```python
from build123d import *

# Parameters (mm, degrees)
F1_DEPTH = 12
F2_DEPTH = 25
F3_R     = 2.5
F4_DEPTH = 25


# Not quite as in the source:
# - a feature names something its author has since deleted; it is built from what else it names


with BuildPart() as f1:
    # F0 (on Top) → F1 (new body)
    with BuildSketch(Plane.XY):
        with BuildLine():
            Line((5, 0), (0, -5))
            Line((0, -5), (0, -30))
            Line((0, -30), (0, -35))
            Line((0, -35), (0, -60))
            Line((0, -60), (0, -65))
            Line((0, -65), (0, -100))
            Line((0, -100), (17.4887780242, -90.9055213439))
            Line((17.4887780242, -90.9055213439), (17.4887780242, -46.2056212127))
            Line((17.4887780242, -46.2056212127), (17.4887780242, -29))
            Line((17.4887780242, -29), (17.4887780242, -20.1109461486))
            Line((17.4887780242, -20.1109461486), (57.2072267532, -20.1109461486))
            Line((57.2072267532, -20.1109461486), (65.1114210486, -29))
            Line((65.1114210486, -29), (132.5, -29))
            ThreePointArc((132.5, -29), (144.1672618896, -24.1672618896), (149, -12.5))
            Line((149, -12.5), (150, 0))
            Line((150, 0), (145.9653675556, 0))
            Line((145.9653675556, 0), (145, -1.1582256993))
            Line((145, -1.1582256993), (145, -3.3333333333))
            Line((145, -3.3333333333), (145, -12.5))
            ThreePointArc((145, -12.5), (132.5, -25), (120, -12.5))
            Line((120, -12.5), (120, -2))
            Line((120, -2), (118, 0))
            Line((118, 0), (97, 0))
            Line((97, 0), (95, -2))
            Line((95, -2), (95, -12.5))
            ThreePointArc((95, -12.5), (82.5, -25), (70, -12.5))
            Line((70, -12.5), (70, -2))
            Line((70, -2), (68, 0))
            Line((68, 0), (5, 0))
        make_face()
    extrude(amount=F1_DEPTH)

    # F0 (on Top) → F2 (cut)
    with BuildSketch(Plane.XY):
        Polygon((17.4887780242, -46.2056212127), (17.4887780242, -90.9055213439), (27.4864036634, -85.7065764627), (108.4292656183, -38.1771444678), (132.5, -29), (65.1114210486, -29), (57.2072267532, -29), (57.2072267532, -46.2056212127), align=None)
    extrude(amount=-F2_DEPTH, mode=Mode.SUBTRACT)

    # F3 (on face) → F4 (cut)
    with BuildSketch(Plane(origin=(0, 0, 0), x_dir=(0, -1, 0), z_dir=(-1, 0, 0))):
        with Locations((25, 6)):
            Circle(F3_R)
        with Locations((50, 6)):
            Circle(F3_R)
    extrude(amount=-F4_DEPTH, mode=Mode.SUBTRACT)


solid = f1.part
```
CAD build for the part. Positions are in the model's coordinates, mm. A direction names the side the tool comes from. Round coordinates to 2 decimals unless told otherwise and drop trailing zeros. Order: outer loops, then holes, each group sorted by start corner. A loop starts at its lowest first (then second) coordinate and runs counter-clockwise, first axis right, second up.
Item 1: Saw through at C-C on y = -11. Write the cut outline in (x, z), then the cut area to 3 significant figures.
Item 2: Pin check, flat tips, straight feed: pin 1 (4 mm diameter, centred on x = 94.5, z = 10, fed in from +Y); pin 2 (2 mm diameter, centred on x = 21, z = 5, fed in from -Y); pin 3 (3 mm diameter, centred on y = -18, z = 7.5, fed in from +X). Stop position of each tip, or through.
Item 3: Probe line 1 along X through (y, z) = (-13, 5); line 2 along X through (y, z) = (-9, 1.75); line 3 along Z through (x, y) = (12.5, -50). List the from-to ranges inside material, lowest first.
Item 4: Mould opens along Z. For faces 1 (the face through (8.622, -52.385, 6.751)), 2 (the face through (144.038, -24.295, 5.916)), 3 (the face through (58, -20, 0)) say: pulls with the +Z half, pulls with the -Z half, needs draft (parallel to the pull), parting line crosses it, or undercut.
Item 5: Saw through at A-A on z = 6. State how many separate pieces and enclosed holes the cut face has, then the cut area to 3 significant figures.
Item 6: Tool access for faces 4 (the face through (8.62, -23.16, 7.69)), 5 (the face through (70, -7, 6)), 6 (the face through (37, -20.111, 6)), 7 (the face through (98, -29, 6)): list every direction of +Z, -Z, +X, -X, +Y, -Y with a clear straight run to the whole face (end or side of a thin tool).
Item 7: Saw through at D-D on x = 108.5. Write the cut outline in (y, z), then the cut area to 3 significant figures.
Item 8: Saw through at B-B on y = -50. Write the cut outline in (x, z), then the cut area to 3 significant figures.
Reported:
1. outline: (0, 0) - (70, 0) - (70, 12) - (0, 12) - close; (95, 0) - (120, 0) - (120, 12) - (95, 12) - close; (145, 0) - (149.12, 0) - (149.12, 12) - (145, 12) - close
1. area: 1,190 mm2
2. pin 1: stops at y = -0.5
2. pin 2: stops at y = -20.11
2. pin 3: stops at x = 148.51
3. line 1: x = 0 to 70.01, 94.99 to 120.01, 144.99 to 148.99
3. line 2: x = 0 to 70, 95 to 120, 145 to 149.28
3. line 3: z = 0 to 3.5, 8.5 to 12
4. face 1: undercut
4. face 2: needs draft
4. face 3: pulls with the -Z half
5. separate pieces: 3
5. enclosed holes: 0
5. area: 3,730 mm2
6. face 4: -X
6. face 5: +Z, -Z, +Y
6. face 6: +Z, -Z, -Y
6. face 7: +Z, -Z, +X, -Y
7. outline: (-29, 0) - (0, 0) - (0, 12) - (-29, 12) - close
7. area: 348 mm2
8. outline: (0, 0) - (17.49, 0) - (17.49, 3.5) - (0, 3.5) - close; (0, 8.5) - (17.49, 8.5) - (17.49, 12) - (0, 12) - close
8. area: 122 mm2
